Drawing for the job (mm, zero at the part's lowest x, y, z). Round coordinates to 2 decimals unless told otherwise and drop trailing zeros. Write each loop counter-clockwise with the first axis right and the second up, starting at its lowest first coordinate (ties: lowest second). Pieces come first, ordered by that corner, then holes. Notation, with made-up numbers: (74, 63) - (129, 63) arc R24 cw to (129, 95) - close; hole circle Ø8 at (46, 67). An arc over 180 degrees is marked (long way). One line per question, with ' | ' between items.
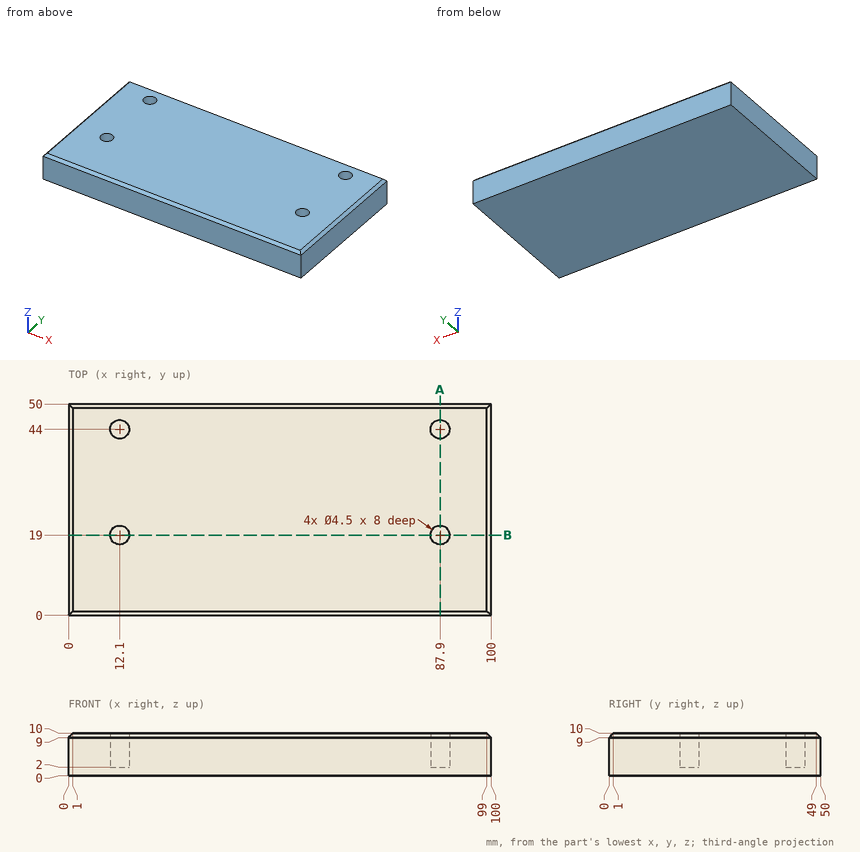
Q1. Saw through at B-B, the plane y = 19. List the corners of the cut face in (x, z).
Found:
outline: (0, 0) - (100, 0) - (100, 9) - (99, 10) - (90.15, 10) - (90.15, 2) - (85.65, 2) - (85.65, 10) - (14.35, 10) - (14.35, 2) - (9.85, 2) - (9.85, 10) - (1, 10) - (0, 9) - close
Q2. Drop a flat-ended pin along its axis: pin 1 (2 mm diameter, centred on x = 89, y = 44, fed in from +Z). Give the stop position or say it passes through.
Found:
pin 1: z = 2
Q3. Saw through at A-A, the plane x = 87.9. List the corners of the cut face in (y, z).
Found:
outline: (0, 0) - (50, 0) - (50, 9) - (49, 10) - (46.25, 10) - (46.25, 2) - (41.75, 2) - (41.75, 10) - (21.25, 10) - (21.25, 2) - (16.75, 2) - (16.75, 10) - (1, 10) - (0, 9) - close
Q4. Drill centre lines: L1, parallel to X at y = 44, z = 6; L2, parallel to Y at x = 87.9, z = 6.5; L3, parallel to X at y = 21, z = 6.25. Where is each one in solid material? Low to high. Write a range as from..to.
Found:
L1: 0..9.85, 14.35..85.65, 90.15..100 | L2: 0..16.75, 21.25..41.75, 46.25..50 | L3: 0..11.07, 13.13..86.87, 88.93..100
